The listing builds one solid part. Answer for the finished solid, in the listing's coordinates (mm). A direction names the side the tool comes from. Coordinates: 2 decimals unless noted, no trailing zeros. Order: outer loops, then holes, each group sorted by start corner. A loop starts at its lowest first (then second) coordinate and runs counter-clockwise, first axis right, second up. Notation, with made-up numbers: (67, 61.25) -> (87, 61.25) arc R18 ccw to (87, 88.25) -> close; hole circle Ø10 at (28.5, 49). An arc over 180 degrees is marked (long way). Answer in a Markdown table with one row per item.
```python
from build123d import *

# Parameters (mm, degrees)
FURO1_D       = 11
FURO1_DEPTH   = 55.7
FURO2_D       = 9.4
FURO2_DEPTH   = 8
FILETE2_R     = 0.5
FILETE3_R     = 0.5
FILETE4_R     = 0.5
CHANFRO1_SIZE = 1


with BuildPart() as part:
    # Esboço1 → Revolução1 (revolve)
    with BuildSketch(Plane.XY, mode=Mode.PRIVATE) as revolu_o1_sk:
        Polygon((0, 0), (63.5, 0), (63.5, 11), (53.5, 11), (53.5, 9.5), (48.5, 9.5), (48.5, 11), (5, 11), (5, 9.5), (0, 9.5), align=None)
    revolve(revolu_o1_sk.sketch.rotate(Axis((0, 0, 0), (1, 0, 0)), 90), axis=Axis((0, 0, 0), (1, 0, 0)))

    # Furo1
    with Locations(Plane(origin=(63.5, 0, 0), x_dir=(0, 0, -1), z_dir=(1, 0, 0))):
        with Locations((0, 0)):
            Hole(FURO1_D / 2, depth=FURO1_DEPTH)

    # Furo2
    with Locations(Plane.ZY):
        with Locations((0, 0)):
            Hole(FURO2_D / 2, depth=FURO2_DEPTH)

    # Filete2
    filete2_edges = [part.edges().sort_by_distance(p)[0] for p in [
        (63.5, 0, -11),
        (53.5, 0, -11),
    ]]
    fillet(filete2_edges, radius=FILETE2_R)

    # Filete3
    filete3_edges = [part.edges().sort_by_distance(p)[0] for p in [
        (0, 0, 4.7),
    ]]
    fillet(filete3_edges, radius=FILETE3_R)

    # Filete4
    filete4_edges = [part.edges().sort_by_distance(p)[0] for p in [
        (0, 0, -9.5),
    ]]
    fillet(filete4_edges, radius=FILETE4_R)

    # Chanfro1
    chanfro1_edges = [part.edges().sort_by_distance(p)[0] for p in [
        (5, 0, -11),
        (48.5, 0, -11),
    ]]
    chamfer(chanfro1_edges, length=CHANFRO1_SIZE)


solid = part.part
```
(1) Find the intervals of material crossed by line 1 along X through (y, z) = (-8, 5.5); line 2 along Y through (x, z) = (21.5, 0); line 3 along Z through (x, y) = (40.5, -0.25), in increasing order. Write a range as from..to.
Check values:
| item | result |
|---|---|
| line 1 | 5..48.5, 53.5..63.5 |
| line 2 | -11..-5.5, 5.5..11 |
| line 3 | -11..-5.49, 5.49..11 |
(2) A cutting plane is placed at A-A, the plane x = 50. Determine the outline of the cut face in (y, z), then the cut area to 3 significant figures.
Check values:
| item | result |
|---|---|
| outline | circle Ø19 at (0, 0); hole circle Ø11 at (0, 0) |
| area | 188 mm² |
(3) Which of the six approach directions +Z, -Z, +X, -X, +Y, -Y give full straight-line access (tool end or side, diameter ignored) to faces 1 (the flat face through (53.5, 9, -5)), 2 (the cylindrical face through (35.26, -5.37, -1.19)), 3 (the flat face through (5, 4, 9)), 4 (the cylindrical face through (58.44, 10.74, -2.38))?
Check values:
| item | result |
|---|---|
| face 1 | none |
| face 2 | +X |
| face 3 | -X |
| face 4 | +X, -X |
(4) A cutting plane is placed at B-B, the plane x = 37.5. Determine the outline of the cut face in (y, z).
Check values:
| item | result |
|---|---|
| outline | circle Ø22 at (0, 0); hole circle Ø11 at (0, 0) |
(5) For a pull along Y with two mould halves and no side action, classify faces 5 (the cylindrical face through (50.965, 9.274, -2.059)), 6 (the cylindrical face through (4.2, -4.59, 1.02)), 7 (the flat face through (63.5, 5, -5)) as released by +Y, released by -Y, zero draft, split by the parting line, or undercut.
Check values:
| item | result |
|---|---|
| face 5 | split by the parting line |
| face 6 | undercut |
| face 7 | zero draft |
(6) Flat-ended cylindrical pins translate along their axes: pin 1 (6 mm diameter, centred on x = 38.5, y = -8, fed in from -Z); pin 2 (1.5 mm diameter, centred on x = 39, y = -5.5, fed in from -Z); pin 3 (8 mm diameter, centred on x = 23.5, y = 8.5, fed in from -Z). Find the tip coordinate at first contact, or state that the pin passes through.
Check values:
| item | result |
|---|---|
| pin 1 | z = -9.8 |
| pin 2 | z = -9.92 |
| pin 3 | z = -10.04 |
